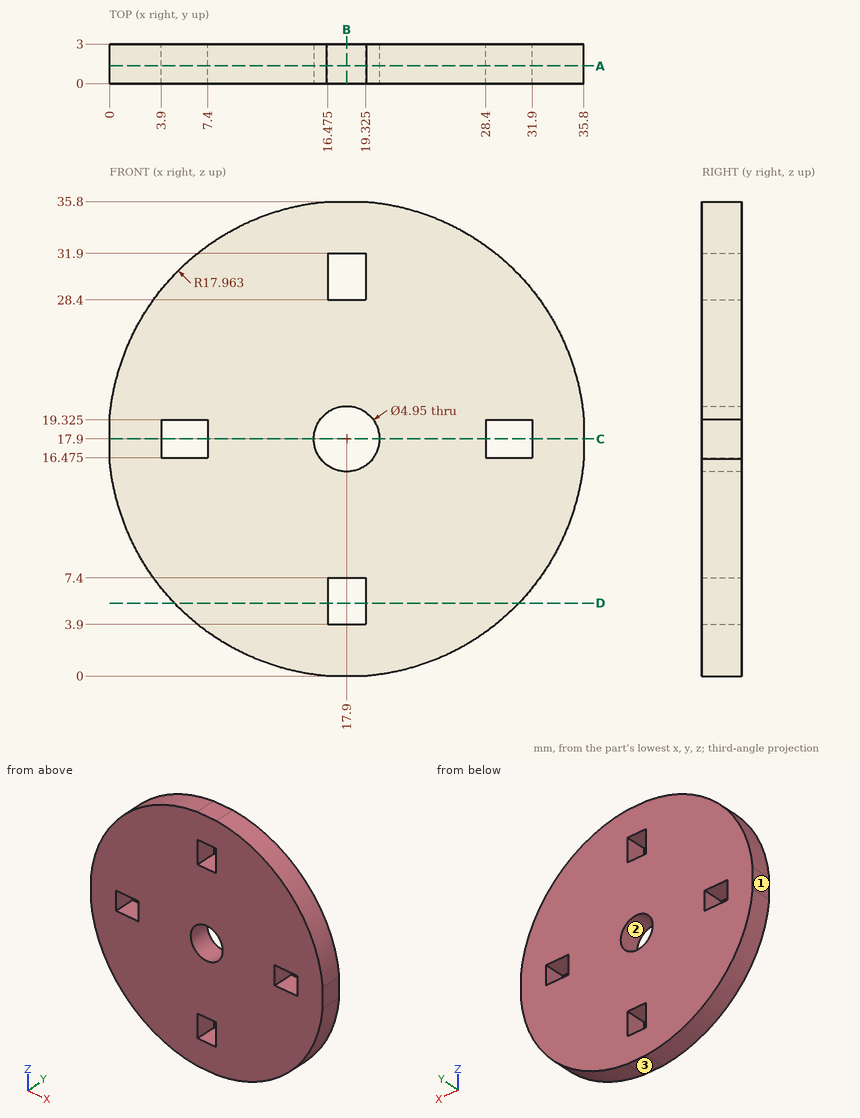
Could you check a few things on this drawing? It's one solid part, dimensions in mm from its lowest x, y, z. Round coordinates to 2 decimals unless told otherwise and drop trailing zeros. Order: outer loops, then holes, each group sorted by start corner. A loop starts at its lowest first (then second) coordinate and runs counter-clockwise, first axis right, second up.
(1) Imagine slicing it at A-A (y = 1.35). Count the separate pieces of the cut face and the enclosed holes in it, plus the area to 3 significant figures.
Response values:
separate pieces: 1
enclosed holes: 5
area: 954 mm2
(2) Imagine slicing it at D-D (z = 5.5). Write out the boundary of the cut face in (x, y) (1 decimal).
Response values:
outline: (4.9, 0) - (16.5, 0) - (16.5, 3) - (4.9, 3) - close; (19.3, 0) - (30.9, 0) - (30.9, 3) - (19.3, 3) - close
(3) Please list where these lines run through material, in increasing order: line 1 along X through (y, z) = (2.3, 17.9) (1 decimal); line 2 along Z through (x, y) = (18.5, 2.7); line 3 along Z through (x, y) = (20, 0.2).
Response values:
line 1: x = 0 to 3.9, 7.4 to 15.4, 20.4 to 28.4, 31.9 to 35.8
line 2: z = 0 to 3.9, 7.4 to 15.5, 20.3 to 28.4, 31.9 to 35.8
line 3: z = 0.06 to 16.59, 19.21 to 35.74
(4) I'm going to push flat-ended pins straight in: pin 1 (1.5 mm diameter, centred on y = 2, z = 5, fed in from -X); pin 2 (0.9 mm diameter, centred on x = 30, y = 1.5, fed in from +Z); pin 3 (0.9 mm diameter, centred on x = 5.5, y = 1.5, fed in from +Z). Where does each tip first touch, or does it pass through?
Response values:
pin 1: stops at x = 4.67
pin 2: stops at z = 31.57
pin 3: stops at z = 31.31
(5) If we mould it in two halves opening along Z, with no side actions, what happens to the marked faces 1, 2 and 3? For each: released by +Z, released by -Z, zero draft, split by the parting line, or undercut.
Response values:
face 1: zero draft
face 2: undercut
face 3: released by -Z
(6) Imagine slicing it at B-B (x = 17.9). Write out the boundary of the cut face in (y, z) (1 decimal).
Response values:
outline: (0, 0) - (3, 0) - (3, 3.9) - (0, 3.9) - close; (0, 7.4) - (3, 7.4) - (3, 15.4) - (0, 15.4) - close; (0, 20.4) - (3, 20.4) - (3, 28.4) - (0, 28.4) - close; (0, 31.9) - (3, 31.9) - (3, 35.8) - (0, 35.8) - close
(7) Imagine slicing it at C-C (z = 17.9). Write out the boundary of the cut face in (x, y) (1 decimal).
Response values:
outline: (0, 0) - (3.9, 0) - (3.9, 3) - (0, 3) - close; (7.4, 0) - (15.4, 0) - (15.4, 3) - (7.4, 3) - close; (20.4, 0) - (28.4, 0) - (28.4, 3) - (20.4, 3) - close; (31.9, 0) - (35.8, 0) - (35.8, 3) - (31.9, 3) - close
